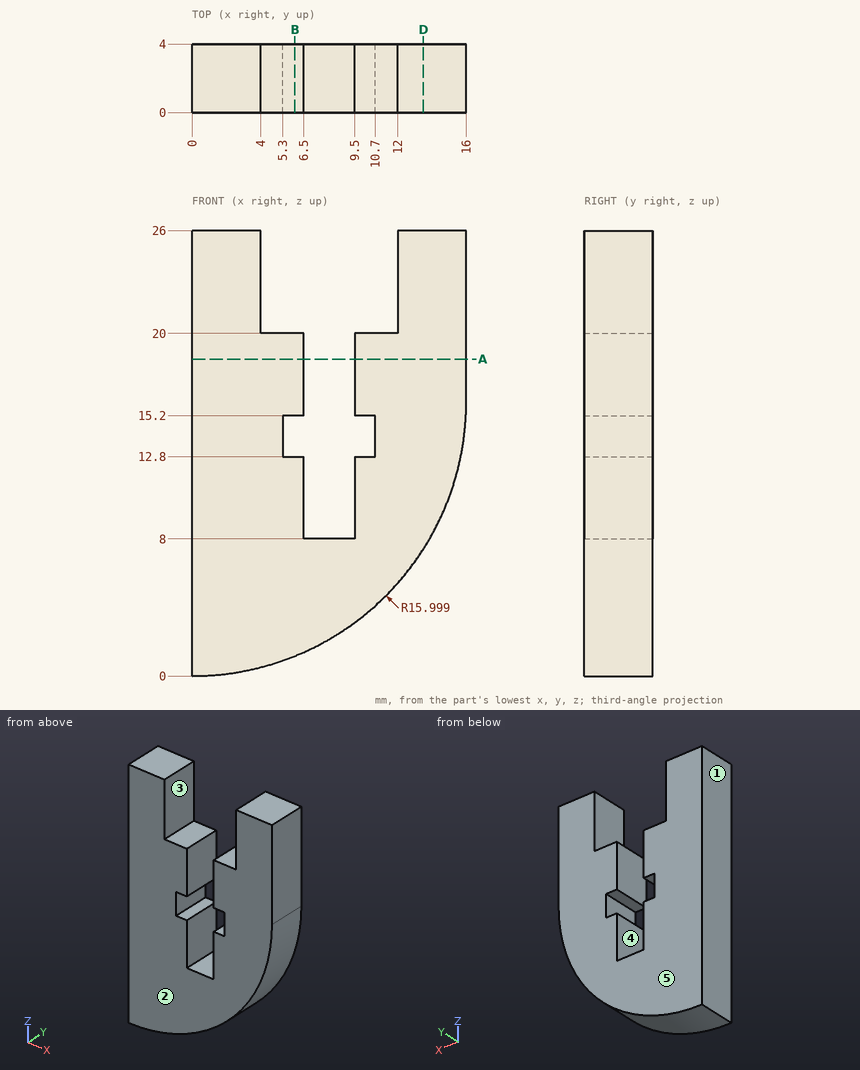
Could you check a few things on this drawing? It's one solid part, dimensions in mm from its lowest x, y, z. A direction names the side the tool comes from. Round coordinates to 2 decimals unless told otherwise and drop trailing zeros. Write each loop counter-clockwise with the first axis right and the second up, starting at its lowest first coordinate (ties: lowest second). Pieces come first, ordered by that corner, then holes.
Q1. Which directions (+Z, -Z, +X, -X, +Y, -Y) give clear straight access to the entire face, cutting with the end or side of a thin tool? Please do the marked faces 4 and 5.
Q2. Please list where these lines run through material, in increasing order: probe 1 along X at (y, z) = (2.75, 23); probe 2 along X at (y, z) = (0.9, 18); probe 3 along Z at (x, y) = (10.5, 0.25) (1 decimal).
Q3. If we section it at A-A on z = 18.5: Write out the boundary of the cut face in (x, y), plus the area to 3 significant figures.
Q4. If we section it at D-D on x = 13.5: Write out the boundary of the cut face in (y, z).
Q5. If we mould it in two halves opening along X, with no side actions, what happens to the marked faces 1, 2 and 3? For each: +X half, -X half, draft (parallel to the pull), parting line (faces both ways), or undercut.
Q6. If we section it at B-B on x = 6: Write out the boundary of the cut face in (y, z).
Q7. Will these pins go through, and if not, where does the flat tip stop? P1, Ø2, axis at y = 3, z = 24, coming from the -X side; P2, Ø0.6, axis at x = 5.5, y = 2, coming from the +Z side; P3, Ø1, axis at y = 3, z = 11, coming from the +X side (1 decimal); P4, Ø0.6, axis at x = 5.5, y = 1.5, coming from the -Z side.
Answer below:
1. face 4: +Z, +Y, -Y
1. face 5: +Z, -Z, +X, -X, +Y
2. probe 1: x = 0 to 4, 12 to 16
2. probe 2: x = 0 to 6.5, 9.5 to 16
2. probe 3: z = 3.9 to 12.8, 15.2 to 20
3. outline: (0, 0) - (6.5, 0) - (6.5, 4) - (0, 4) - close; (9.5, 0) - (16, 0) - (16, 4) - (9.5, 4) - close
3. area: 52.0 mm2
4. outline: (0, 7.41) - (4, 7.41) - (4, 26) - (0, 26) - close
5. face 1: -X half
5. face 2: draft
5. face 3: undercut
6. outline: (0, 1.17) - (4, 1.17) - (4, 12.8) - (0, 12.8) - close; (0, 15.2) - (4, 15.2) - (4, 20) - (0, 20) - close
7. P1: stops at x = 0
7. P2: stops at z = 20
7. P3: stops at x = 15.4
7. P4: stops at z = 0.87
